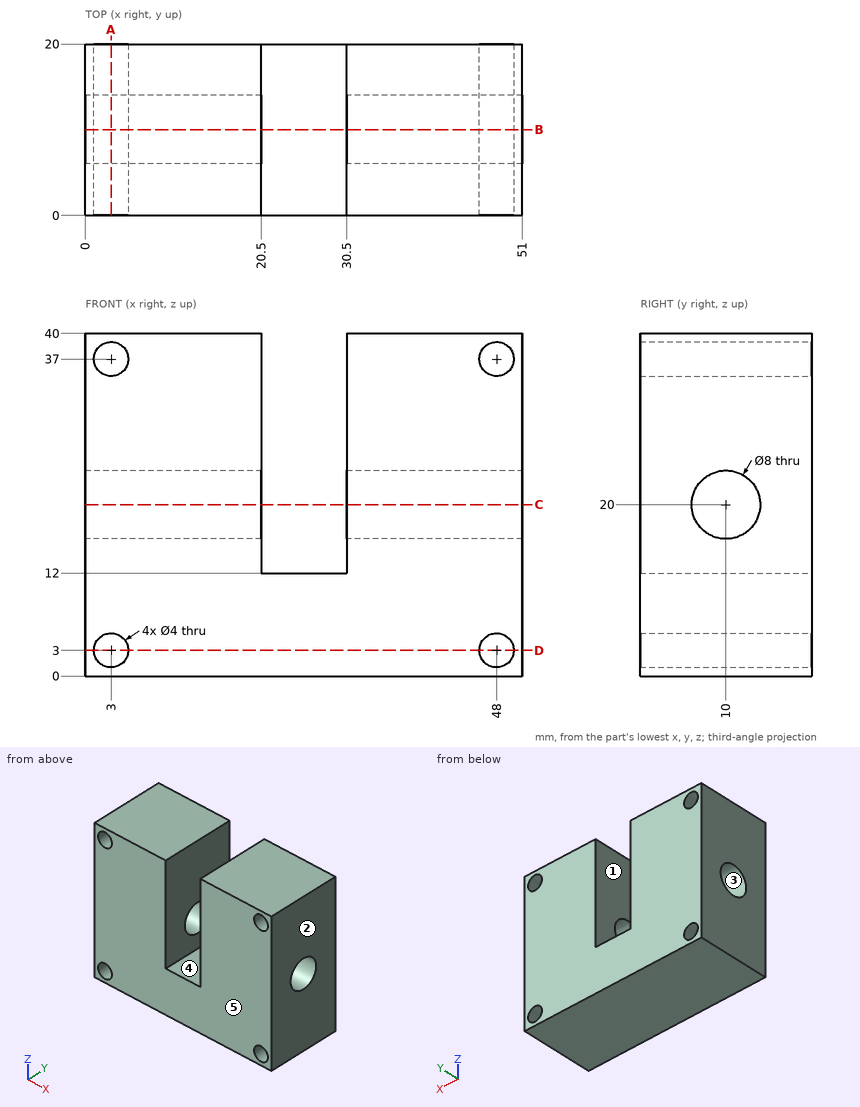
The drawing under review shows one solid part. Ordinate dimensions are in mm from its lowest x, y, z. A direction names the side the tool comes from. Round coordinates to 2 decimals unless told otherwise and drop trailing zeros. Loops run counter-clockwise (first coordinate to the right, second up) from the corner with the lowest first, then second, coordinate; pieces in that order, holes last. Notation, with made-up numbers: (-13, -16) -> (-3, -16) arc R25 ccw to (-3, 22) -> close; hole circle Ø4 at (-25.5, 54). An arc over 180 degrees is marked (long way). Answer in a Markdown table with one row per item.
1) Wall thickness on line 1 along X through (y, z) = (12.75, 37); line 2 along X through (y, z) = (11.5, 3); line 3 along X through (y, z) = (7.5, 29): over which ranges is each line inside the solid? List them lowest first.
Taken from the geometry:
| item | result |
|---|---|
| line 1 | x = 0 to 1, 5 to 20.5, 30.5 to 46, 50 to 51 |
| line 2 | x = 0 to 1, 5 to 46, 50 to 51 |
| line 3 | x = 0 to 20.5, 30.5 to 51 |
2) Tool access review of the marked faces 4 and 5: name each direction out of +Z, -Z, +X, -X, +Y, -Y from which nothing blocks a thin tool from reaching the whole face with its end or side.
Taken from the geometry:
| item | result |
|---|---|
| face 4 | +Z, +Y, -Y |
| face 5 | +Z, -Z, +X, -X, -Y |
3) Draft analysis for pull direction X (two halves, no side actions). For the marked faces 1, 2 and 3, state which applies: pulls with the +X half, pulls with the -X half, needs draft (parallel to the pull), parting line crosses it, or undercut.
Taken from the geometry:
| item | result |
|---|---|
| face 1 | undercut |
| face 2 | pulls with the +X half |
| face 3 | needs draft |
4) For pin 1 Ø8 at (y, z) = (17, 22.5) entering from -X; pin 2 Ø8 at (x, y) = (25, 11.5) entering from +Z, all flat-tipped, find the tip position at first contact; note any pin that passes through.
Taken from the geometry:
| item | result |
|---|---|
| pin 1 | stops at x = 0 |
| pin 2 | stops at z = 12 |
5) Consider section C-C, the plane z = 20. Write out the cut boundary in (x, y), plus the area to 3 significant figures.
Taken from the geometry:
| item | result |
|---|---|
| outline | (0, 0) -> (20.5, 0) -> (20.5, 6) -> (0, 6) -> close; (0, 14) -> (20.5, 14) -> (20.5, 20) -> (0, 20) -> close; (30.5, 0) -> (51, 0) -> (51, 6) -> (30.5, 6) -> close; (30.5, 14) -> (51, 14) -> (51, 20) -> (30.5, 20) -> close |
| area | 492 mm² |
6) Consider section B-B, the plane y = 10. Write out the cut boundary in (x, z).
Taken from the geometry:
| item | result |
|---|---|
| outline | (0, 0) -> (51, 0) -> (51, 16) -> (30.5, 16) -> (30.5, 12) -> (20.5, 12) -> (20.5, 16) -> (0, 16) -> close; (0, 24) -> (20.5, 24) -> (20.5, 40) -> (0, 40) -> close; (30.5, 24) -> (51, 24) -> (51, 40) -> (30.5, 40) -> close; hole circle Ø4 at (3, 3); hole circle Ø4 at (3, 37); hole circle Ø4 at (48, 3); hole circle Ø4 at (48, 37) |
7) Consider section A-A, the plane x = 3. Write out the cut boundary in (y, z).
Taken from the geometry:
| item | result |
|---|---|
| outline | (0, 0) -> (20, 0) -> (20, 1) -> (0, 1) -> close; (0, 5) -> (20, 5) -> (20, 35) -> (0, 35) -> close; (0, 39) -> (20, 39) -> (20, 40) -> (0, 40) -> close; hole circle Ø8 at (10, 20) |
8) Consider section D-D, the plane z = 3. Write out the cut boundary in (x, y), plus the area to 3 significant figures.
Taken from the geometry:
| item | result |
|---|---|
| outline | (0, 0) -> (1, 0) -> (1, 20) -> (0, 20) -> close; (5, 0) -> (46, 0) -> (46, 20) -> (5, 20) -> close; (50, 0) -> (51, 0) -> (51, 20) -> (50, 20) -> close |
| area | 860 mm² |
